Read the model definition and answer for the solid it produces. Units are mm, in the model's axes. Coordinates: 2 decimals unless noted, no trailing zeros. Loops run counter-clockwise (first coordinate to the right, second up) from the corner with the lowest first, then second, coordinate; pieces in that order, holes last. Notation, with made-up numbers: M 44,46.25 L 78,46.25 A32 ccw 78,72.25 Z; hole C 58.5,17.25 d6. An arc over 180 degrees is marked long. Use one line per item in the form item = value. Start each with the question number.
1. The part is cut by section A-A (x = 3.5). Give the vertices of the cut face in (y, z).
2. The part is cut by section B-B (z = 12.25). Give the number of separate pieces and of enclosed holes in the cut face, plus the area to 3 significant figures.
3. Find the intervals of material crossed by probe 1 along Y at (x, z) = (-15.5, 7); probe 2 along Z at (x, y) = (-11, 1.75); probe 3 along Y at (x, z) = (-11, 9), in increasing order. Write a range as [from, to].
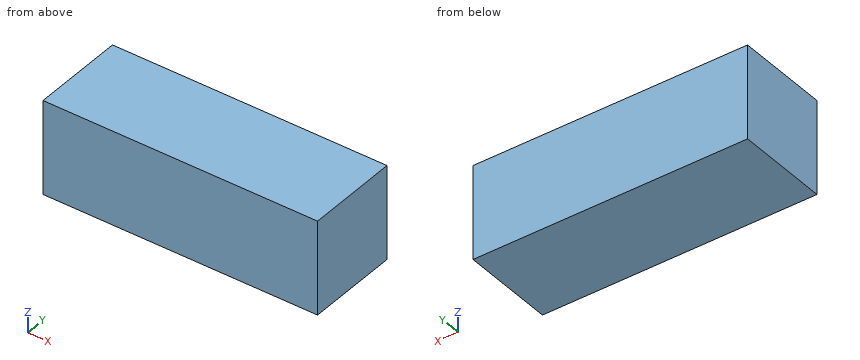
from build123d import *

# Parameters (mm, degrees)
F0_W     = 41
F0_H     = 14
F1_DEPTH = 1
F2_W     = 41
F2_H     = 14
F2_W_2   = 39
F2_H_2   = 12
F3_DEPTH = 12
F2_R     = 0.75
F4_DEPTH = 12
F5_W     = 41
F5_H     = 14
F6_DEPTH = 1


with BuildPart() as f1:
    # F0 (on Top) → F1 (new body)
    with BuildSketch(Plane.XY):
        Rectangle(F0_W, F0_H)
    extrude(amount=F1_DEPTH)

    # F2 (on face) → F3 (join)
    with BuildSketch(Plane.XY.offset(1)):
        Rectangle(F2_W, F2_H)
        Rectangle(F2_W_2, F2_H_2, mode=Mode.SUBTRACT)
    extrude(amount=F3_DEPTH)

    # F2 (on face) → F4 (join)
    with BuildSketch(Plane.XY.offset(1)):
        Rectangle(F2_W_2, F2_H_2)
        with Locations((-15.5, -2)):
            Circle(F2_R, mode=Mode.SUBTRACT)
        with Locations((-11.5, -2)):
            Circle(F2_R, mode=Mode.SUBTRACT)
        with Locations((-7.5, -2)):
            Circle(F2_R, mode=Mode.SUBTRACT)
        with Locations((-3.5, -2)):
            Circle(F2_R, mode=Mode.SUBTRACT)
        with Locations((3.5, -2)):
            Circle(F2_R, mode=Mode.SUBTRACT)
        with Locations((7.5, -2)):
            Circle(F2_R, mode=Mode.SUBTRACT)
        with Locations((11.5, -2)):
            Circle(F2_R, mode=Mode.SUBTRACT)
        with Locations((15.5, -2)):
            Circle(F2_R, mode=Mode.SUBTRACT)
        with Locations((-15.5, 2)):
            Circle(F2_R, mode=Mode.SUBTRACT)
        with Locations((-11.5, 2)):
            Circle(F2_R, mode=Mode.SUBTRACT)
        with Locations((-7.5, 2)):
            Circle(F2_R, mode=Mode.SUBTRACT)
        with Locations((-3.5, 2)):
            Circle(F2_R, mode=Mode.SUBTRACT)
        with Locations((3.5, 2)):
            Circle(F2_R, mode=Mode.SUBTRACT)
        with Locations((7.5, 2)):
            Circle(F2_R, mode=Mode.SUBTRACT)
        with Locations((11.5, 2)):
            Circle(F2_R, mode=Mode.SUBTRACT)
        with Locations((15.5, 2)):
            Circle(F2_R, mode=Mode.SUBTRACT)
    extrude(amount=F4_DEPTH)

    # F5 (on face) → F6 (join)
    with BuildSketch(Plane.XY.offset(13)):
        Rectangle(F5_W, F5_H)
    extrude(amount=F6_DEPTH)


solid = f1.part
Computed values:
q1.outline = M -7,0 L 7,0 L 7,14 L -7,14 Z; hole M -2.75,1 L -1.25,1 L -1.25,13 L -2.75,13 Z; hole M 1.25,1 L 2.75,1 L 2.75,13 L 1.25,13 Z
q2.separate_pieces = 1
q2.enclosed_holes = 16
q2.area = 546 mm²
q3.probe_1 = [-7, -2.75], [-1.25, 1.25], [2.75, 7]
q3.probe_2 = [0, 1], [13, 14]
q3.probe_3 = [-7, -2.56], [-1.44, 1.44], [2.56, 7]
